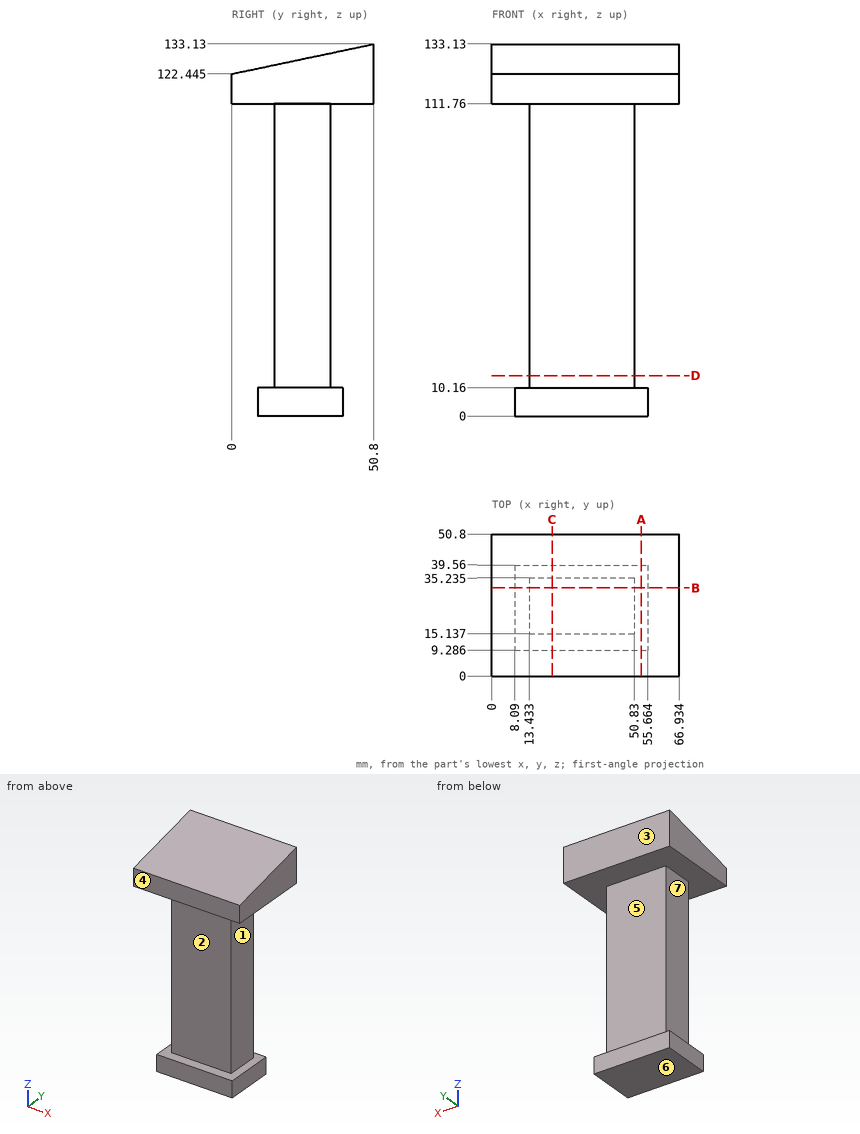
Job drawing, mm, ordinate dimensions from the low corner. One solid piece. A direction names the side the tool comes from. Round coordinates to 2 decimals unless told otherwise and drop trailing zeros. Order: outer loops, then holes, each group sorted by start corner. A loop starts at its lowest first (then second) coordinate and runs counter-clockwise, first axis right, second up. Notation, with made-up numbers: (33.25, -4) -> (51.25, -4) arc R7 ccw to (51.25, 4) -> close; hole circle Ø2 at (25, -6.75). An arc over 180 degrees is marked (long way). Write item = value, one per line.
(1) Pull direction Z, two halves, no side cores. Call the marked faces 4, 5, 6 and 7: +Z half, -Z half, draft (parallel to the pull), parting line (faces both ways), or undercut.
Answers follow:
face_4 = draft
face_5 = undercut
face_6 = -Z half
face_7 = undercut
(2) 3-axis set-ups, long thin cutter, end or side, ignore diameter. For the marked faces 1, 2 and 3: which of +Z, -Z, +X, -X, +Y, -Y reach the whole face in a straight line?
Answers follow:
face_1 = +X, +Y, -Y
face_2 = +X, -X, -Y
face_3 = +Z, -Z, +X, -X, +Y
(3) Cut at A-A (x = 53.5). Write the cut outline in (y, z) (1 decimal).
Answers follow:
outline = (0, 111.8) -> (50.8, 111.8) -> (50.8, 133.1) -> (0, 122.4) -> close; (9.3, 0) -> (39.6, 0) -> (39.6, 10.2) -> (9.3, 10.2) -> close
(4) Flat gauge pins, fed straight in: P1, Ø3, axis at x = 12.5, z = 105.5, coming from the -Y side; P2, Ø8, axis at x = 41.5, z = 7, coming from the +Y side; P3, Ø8, axis at y = 25, z = 5.5, coming from the -X side. Where does each tip first touch, or does it go through?
Answers follow:
P1 = 15.14
P2 = 39.56
P3 = 8.09
(5) Drill centre lines: L1, parallel to Y at x = 33.5, z = 24.5 (1 decimal); L2, parallel to X at y = 15.5, z = 104; L3, parallel to Z at x = 33.5, y = 6. Where is each one in solid material? Low to high.
Answers follow:
L1 = 15.1 to 35.2
L2 = 13.43 to 50.83
L3 = 111.76 to 123.71
(6) Cut at D-D (z = 14.5). Write the cut outline in (x, y) (1 decimal).
Answers follow:
outline = (13.4, 15.1) -> (50.8, 15.1) -> (50.8, 35.2) -> (13.4, 35.2) -> close
(7) Cut at B-B (y = 31.5). Write the cut outline in (x, z), plus the area to 3 significant figures.
Answers follow:
outline = (0, 111.76) -> (13.43, 111.76) -> (13.43, 10.16) -> (8.09, 10.16) -> (8.09, 0) -> (55.66, 0) -> (55.66, 10.16) -> (50.83, 10.16) -> (50.83, 111.76) -> (66.93, 111.76) -> (66.93, 129.07) -> (0, 129.07) -> close
area = 5,440 mm²
(8) Cut at C-C (x = 21.5). Write the cut outline in (y, z) (1 decimal), plus the area to 3 significant figures.
Answers follow:
outline = (0, 111.8) -> (15.1, 111.8) -> (15.1, 10.2) -> (9.3, 10.2) -> (9.3, 0) -> (39.6, 0) -> (39.6, 10.2) -> (35.2, 10.2) -> (35.2, 111.8) -> (50.8, 111.8) -> (50.8, 133.1) -> (0, 122.4) -> close
area = 3,160 mm²
